The listing builds one solid part. Answer for the finished solid, in the listing's coordinates (mm). Face numbers are marked on the shaded views. Coordinates: 2 decimals unless noted, no trailing zeros. Order: outer loops, then holes, each group sorted by start corner. A loop starts at its lowest first (then second) coordinate and runs counter-clockwise, first axis right, second up. Notation, with made-up numbers: (2.5, 5) - (54.5, 5) arc R6 ccw to (54.5, 14) - close; hole circle Ø11 at (47, 71). An arc over 180 degrees is marked (long way). Use a Markdown table: item, result. Add a question column.
Item 1: The part is cut by section B-B, the plane z = 5. Give the vertices of the cut face in (x, y), then the cut area to 3 significant figures.
Item 2: Find the intervals of material crossed by line 1 along Z through (x, y) = (-47, -8); line 2 along X through (y, z) = (7.25, -1); line 3 along X through (y, z) = (0.75, 34.5), in increasing order.
Item 3: The part is cut by section D-D, the plane x = 33. Give the vertices of the cut face in (y, z), then the cut area to 3 significant figures.
Item 4: The mould has two halves that part along X. Classify the marked faces 1 and 2: released by +X, released by -X, zero draft, split by the parting line, or undercut.
Item 5: The part is cut by section A-A, the plane z = 51.5. Give the vertices of the cut face in (x, y), then the cut area to 3 significant figures.
Item 6: The part is cut by section C-C, the plane y = 3.25. Give the vertices of the cut face in (x, z), then the cut area to 3 significant figures.
Item 7: Flat-ended cylindrical pins translate along their axes: P1, Ø5.5, axis at x = 61, y = 3, coming from the -Z side; P2, Ø2, axis at y = -5.5, z = 12, coming from the -X side; P3, Ø8, axis at y = 3.5, z = 42, coming from the +X side. Find the tip coordinate at first contact, or state that the pin passes through.
from build123d import *

# Parameters (mm, degrees)
SKETCH2_W            = 20
SKETCH2_H            = 5
M4_CLEARANCE_HOLE1_D = 4.5


with BuildPart() as part:
    # Sweep1: sweep along a path in Sketch1
    with BuildLine(Plane(origin=(0, 0, 0), x_dir=(1, 0, 0), z_dir=(0, 1, 0))) as sweep1_path:
        ThreePointArc((-42.426406871, 42.426406871), (-22.961005942, -55.432771951), (60, 0))
    # Sketch2 → Sweep1 (sweep)
    with BuildSketch(Plane(origin=(0, 0, 0), x_dir=(0, 1, 0), z_dir=(0, 0, 1))):
        with Locations((0, 60)):
            Rectangle(SKETCH2_W, SKETCH2_H)
    sweep(path=sweep1_path.line)

    # M4 Clearance Hole1 (through all)
    with Locations(Plane(origin=(0, -10, 0), x_dir=(-1, 0, 0), z_dir=(0, -1, 0))):
        with Locations((-59.791303716, -5), (45.814370219, 38.743302407)):
            Hole(M4_CLEARANCE_HOLE1_D / 2)


solid = part.part
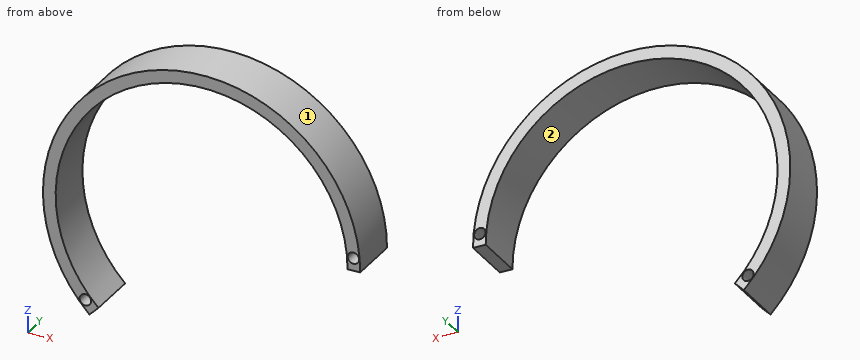
Solution:
| question | item | result |
|---|---|---|
| 1 | outline | (-62.3, -10) - (-57.28, -10) - (-57.28, 10) - (-62.3, 10) - close; (57.28, -10) - (57.54, -10) - (57.54, 10) - (57.28, 10) - close; (62.04, -10) - (62.3, -10) - (62.3, 10) - (62.04, 10) - close |
| 1 | area | 111 mm2 |
| 2 | line 1 | z = -41.2 to -40.66, -36.83 to -33.12, 33.12 to 41.2 |
| 2 | line 2 | x = -62.49 to -57.49 |
| 2 | line 3 | x = -52.12 to -46, 46 to 52.12 |
| 3 | outline | (-10, 47.09) - (10, 47.09) - (10, 53.08) - (-10, 53.08) - close |
| 3 | area | 120 mm2 |
| 4 | face 1 | split by the parting line |
| 4 | face 2 | undercut |
| 5 | outline | (-35.41, -10) - (-25.57, -10) - (-25.57, 10) - (-35.41, 10) - close; (25.57, -10) - (35.41, -10) - (35.41, 10) - (25.57, 10) - close |
| 5 | area | 394 mm2 |
| 6 | outline | (-44.19, -44.19) - (-40.66, -40.66) arc R57.5 cw (long way) to (57.5, 0) - (62.5, 0) arc R62.5 ccw (long way) to start; hole circle Ø4.5 at (-45.81, -38.74); hole circle Ø4.5 at (59.79, 5) |
| 6 | area | 1,150 mm2 |
| 7 | P1 | stops at z = 0 |
| 7 | P2 | stops at x = -61.52 |
| 7 | P3 | stops at x = 49.62 |
